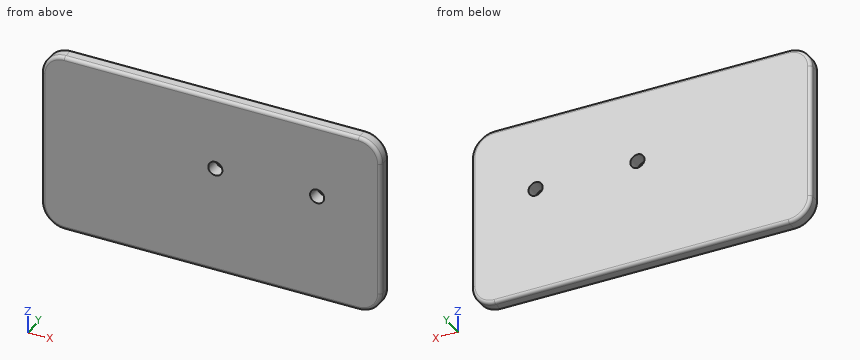
```python
from build123d import *

# Parameters (mm, degrees)
F0_W     = 76.2
F0_H     = 40.64
F0_R     = 1.5875
F1_DEPTH = 3.175
F2_R     = 5.08
F3_R     = 0.762


# Not quite as in the source:
# - a feature names something its author has since deleted; it is built from what else it names


with BuildPart() as f1:
    # F0 (on Front) → F1 (new body)
    with BuildSketch(Plane.XZ):
        with Locations((-5.08, -3.81)):
            Rectangle(F0_W, F0_H)
        with Locations((-4.191, 0)):
            Circle(F0_R, mode=Mode.SUBTRACT)
        with Locations((18.669, 0)):
            Circle(F0_R, mode=Mode.SUBTRACT)
    extrude(amount=F1_DEPTH)

    # F2
    f2_edges = [f1.edges().sort_by_distance(p)[0] for p in [
        (-43.18, -1.5875, -24.13),
        (33.02, -1.5875, 16.51),
        (33.02, -1.5875, -24.13),
        (-43.18, -1.5875, 16.51),
    ]]
    fillet(f2_edges, radius=F2_R)

    # F3
    f3_edges = [f1.edges().sort_by_distance(p)[0] for p in [
        (-5.08, 0, -24.13),
        (-5.08, -3.175, -24.13),
        (-43.18, -3.175, -3.81),
        (-43.18, 0, -3.81),
        (-41.692102, 0, -22.642102),
        (31.532102, 0, -22.642102),
        (33.02, 0, -3.81),
        (-41.692102, 0, 15.022102),
        (31.532102, 0, 15.022102),
        (-5.08, 0, 16.51),
        (-41.692102, -3.175, -22.642102),
        (31.532102, -3.175, -22.642102),
        (33.02, -3.175, -3.81),
        (-41.692102, -3.175, 15.022102),
        (31.532102, -3.175, 15.022102),
        (-5.08, -3.175, 16.51),
    ]]
    fillet(f3_edges, radius=F3_R)


solid = f1.part
```
Source: CAD feature listing. Evaluate the final solid. Frame: model axes, mm. Round coordinates to 2 decimals unless told otherwise and drop trailing zeros. Loops run counter-clockwise (first coordinate to the right, second up) from the corner with the lowest first, then second, coordinate; pieces in that order, holes last. Notation, with made-up numbers: M 87,-17.5 L 91,-17.5 A9 cw 91,-1.5 Z; hole C 37,77.25 d8. An arc over 180 degrees is marked long. Put each result on its own line as item: value.
(1) First-contact query: pin 1 (2.5 mm diameter, centred on x = -4.191, z = 0, fed in from -Y). Flat tip, straight axial feed; report the tip coordinate or a pass-through.
Solutions:
pin 1: through
(2) Section B-B, the plane x = 19. Return loops of the section in (y, z) (3 decimals), and give its area (3 significant figures).
Solutions:
outline: M -3.175,-23.368 A0.762 ccw -2.413,-24.13 L -0.762,-24.13 A0.762 ccw 0,-23.368 L 0,-1.553 L -3.175,-1.553 Z; M -3.175,1.553 L 0,1.553 L 0,15.748 A0.762 ccw -0.762,16.51 L -2.413,16.51 A0.762 ccw -3.175,15.748 Z
area: 119 mm²
(3) Section A-A, the plane z = 0. Return loops of the section in (x, y) (1 decimal).
Solutions:
outline: M -43.2,-2.4 A0.8 ccw -42.4,-3.2 L -5.8,-3.2 L -5.8,0 L -42.4,0 A0.8 ccw -43.2,-0.8 Z; M -2.6,-3.2 L 17.1,-3.2 L 17.1,0 L -2.6,0 Z; M 20.3,-3.2 L 32.3,-3.2 A0.8 ccw 33,-2.4 L 33,-0.8 A0.8 ccw 32.3,0 L 20.3,0 Z
(4) Ray query, line 1 (Z direction, x = -4.5, y = -0.25); line 2 (X direction, y = -2.7, z = 14); line 3 (Z direction, x = -31, y = -2.8). Return the intervals inside material, ascending. Write a range as [from, to].
Solutions:
line 1: [-23.93, -1.56], [1.56, 16.31]
line 2: [-42.42, 32.26]
line 3: [-24.02, 16.4]
